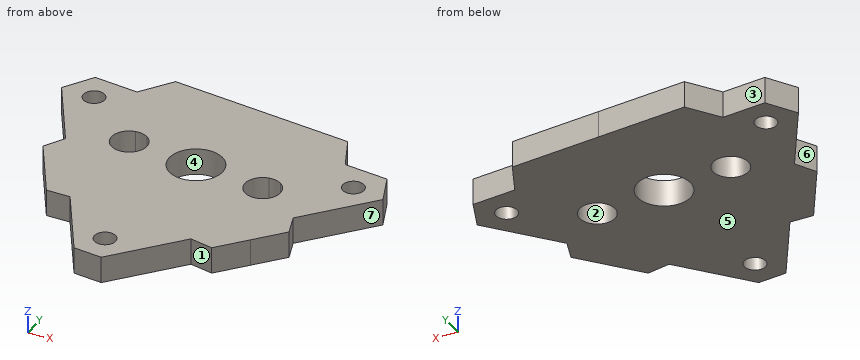
Autodesk Inventor part; units mm, degrees
ref_plane "YZ Plane" through (0, 0, 0) normal (1, 0, 0) x (0, 1, 0)
ref_plane "XZ Plane" through (0, 0, 0) normal (0, 1, 0) x (-1, 0, 0)
ref_plane "XY Plane" through (0, 0, 0) normal (0, 0, 1) x (1, 0, 0)
sketch "Sketch1" plane through (0, 0, 0) normal (0, 0, 1) x (1, 0, 0)
  circle A0 centre (-29.1799, 3.0736) radius 3.175 construction
  circle A1 centre (1.7526, 0) radius 3.175 construction
  circle A2 centre (-15.8567, -20.0304) radius 3.175 construction
  circle A3 centre (-29.1799, 3.0736) radius 1.2
  circle A4 centre (1.7526, 0) radius 1.2
  circle A5 centre (-15.8567, -20.0304) radius 1.2
  line L0 (-29.1799, 3.0736) -> (1.7526, 0) construction
  line L1 (-13.7137, 1.5368) -> (-15.8567, -20.0304) construction
  line L2 (-30.7954, 6.4247) -> (3.9959, 2.9677)
  line L3 (3.9959, 2.9677) -> (5.4173, -0.6401)
  line L4 (5.4173, -0.6401) -> (-14.5484, -23.3511)
  line L5 (-14.5484, -23.3511) -> (-17.7927, -23.0287)
  line L6 (-17.7927, -23.0287) -> (-32.899, 3.1671)
  line L7 (-32.899, 3.1671) -> (-30.7954, 6.4247)
  point P0 (0, 0)
  point P1 (-16.1706, -23.1899)
  point P2 (-31.8472, 4.7959)
  dimension "d0" = 2.4
  dimension "d1" = 2.4
  dimension "d2" = 2.4
extrude "Plate1" add sketch "Sketch1" along normal blind 3
sketch "Sketch2" plane through (0, 0, 3) normal (0, 0, 1) x (1, 0, 0)
  line L0 (-17.7927, -23.0287) -> (-32.899, 3.1671) construction
  line L1 (-30.7954, 6.4247) -> (3.9959, 2.9677) construction
  line L2 (5.4173, -0.6401) -> (-14.5484, -23.3511) construction
  line L3 (-17.7927, -23.0287) -> (-32.899, 3.1671) construction
  line L4 (-25.3459, -9.9308) -> (-14.2154, -3.5122) construction
  line L5 (-14.2154, -3.5122) -> (-13.3997, 4.6962) construction
  line L6 (-14.2154, -3.5122) -> (-4.5656, -11.9956) construction
  line L7 (5.4173, -0.6401) -> (-14.5484, -23.3511) construction
  point P0 (0, 0)
sketch "Sketch3" plane through (0, 0, 3) normal (0, 0, 1) x (1, 0, 0)
  arc A0 (-5.0898, -2.6774) -> (-6.5829, -2.3304) centre (-6.2546, -4.3032) ccw
  arc A1 (-6.5829, -2.3304) -> (-5.0898, -2.6774) centre (-6.2546, -4.3032) ccw
  arc A2 (-21.0113, -1.0954) -> (-22.5045, -0.7484) centre (-22.1762, -2.7212) ccw
  arc A3 (-22.5045, -0.7484) -> (-21.0113, -1.0954) centre (-22.1762, -2.7212) ccw
  circle A4 centre (-14.2154, -3.5122) radius 3
extrude "Extrusion1" cut sketch "Sketch3" against normal through all
sketch "Sketch4" plane through (0, 0, 0) normal (0, 0, -1) x (-1, 0, 0)
  line L0 (30.7954, 6.4247) -> (-3.9959, 2.9677)
  line L1 (0.9857, 3.4627) -> (2.77, 7.4096)
  line L2 (2.77, 7.4096) -> (13.0288, 8.429)
  line L3 (13.0288, 8.429) -> (13.3997, 4.6962) construction
  arc A0 (9.3955, 4.3921) -> (1.4831, 3.2621) centre (5.4635, 3.6576) ccw construction
  line L4 (25.8137, 5.9297) -> (23.2877, 9.4483)
  line L5 (23.2877, 9.4483) -> (13.0288, 8.429)
  line L6 (-5.4173, -0.6401) -> (14.5484, -23.3511)
  line L7 (0.9442, -7.8763) -> (0.0881, -10.4082)
  line L8 (0.0881, -10.4082) -> (2.8272, -13.5239)
  line L9 (2.8272, -13.5239) -> (4.5656, -11.9956) construction
  line L10 (-5.4173, -0.6401) -> (14.5484, -23.3511)
  arc A1 (3.0652, -12.6595) -> (11.0452, -12.2104) centre (7.0456, -12.264) ccw construction
  line L11 (8.1869, -16.1149) -> (5.5662, -16.6395)
  line L12 (5.5662, -16.6395) -> (2.8272, -13.5239)
  line L13 (17.7927, -23.0287) -> (32.899, 3.1671)
  line L14 (28.0858, -5.1794) -> (29.4234, -7.4934)
  line L15 (29.4234, -7.4934) -> (27.351, -11.0871)
  line L16 (25.2786, -14.6808) -> (27.351, -11.0871)
  line L17 (22.6059, -14.6822) -> (25.2786, -14.6808)
  point P0 (0, 0)
  dimension "d6" = 120
  dimension "d7" = 120
extrude "Extrusion2" add sketch "Sketch4" against normal up to surface (3 mm away)
equation "\"d3\" = Thickness"
equation "\"BendRadius\" = Thickness"
equation "\"BendReliefWidth\" = Thickness"
equation "\"BendReliefDepth\" = 0.5 * Thickness"
equation "\"CornerReliefSize\" = 4 * Thickness"
equation "\"MinimumRemnant\" = 2 * Thickness"
equation "\"TransitionRadius\" = BendRadius"
equation "\"JacobiRadiusSize\" = BendRadius"
equation "\"GapSize\" = Thickness"
properties part number "TongueMount"
Here's how the part is built. I have some questions about the finished solid (model axes, mm). Face numbers are marked on the shaded views. A direction names the side the tool comes from. Give positions to 0.01 mm unless a question says otherwise; leave off trailing zeros. Loops run counter-clockwise (first coordinate to the right, second up) from the corner with the lowest first, then second, coordinate; pieces in that order, holes last. Notation, with made-up numbers: (18, 65) -> (69, 65) arc R13 ccw to (69, 85) -> close; hole circle Ø10 at (27, 77). An arc over 180 degrees is marked (long way). Use one line per item in the form item = value. Start each with the question number.
1) Imagine slicing it at C-C (x = 1). Please give me the cut outline in (y, z), then the cut area to 3 significant figures.
2) Thinking about a two-plate mould opening in X: for the marked faces 4, 5, 6 and 7, which applies, +X half, -X half, draft (parallel to the pull), parting line (faces both ways), or undercut?
3) Imagine slicing it at A-A (y = 0). Please give me the cut outline in (x, z).
4) Which directions (+Z, -Z, +X, -X, +Y, -Y) give clear straight access to the entire face, cutting with the end or side of a thin tool? Please do the marked faces 1, 2 and 3.
5) Imagine slicing it at B-B (z = 0.9). Please give me the cut outline in (x, y).
6) Please list where these lines run through material, in increasing order: line 1 along Y through (x, z) = (-15.5, 2); line 2 along X through (y, z) = (-2.5, 0.2); line 3 along X through (y, z) = (-4.5, 1.15).
7) For P1, Ø1, axis at x = -18.5, z = 2.5, coming from the -Y side; P2, Ø5, axis at x = -22.18, y = -2.72, coming from the +Z side; P3, Ø1.9, axis at x = 1.75, y = 0, coming from the +Z side, each with a flat end and sliding along its axis, tell me the tip position at first contact or that it passes through.
8) Imagine slicing it at D-D (y = 7). Please give me the cut outline in (x, z), then the cut area to 3 significant figures.
Check values:
q1.outline = (-5.66, 0) -> (-0.93, 0) -> (-0.93, 3) -> (-5.66, 3) -> close; (0.93, 0) -> (3.27, 0) -> (3.27, 3) -> (0.93, 3) -> close
q1.area = 21.2 mm^2
q2.face_4 = undercut
q2.face_5 = draft
q2.face_6 = -X half
q2.face_7 = +X half
q3.outline = (-31.07, 0) -> (0.55, 0) -> (0.55, 3) -> (-31.07, 3) -> close; (2.95, 0) -> (5.17, 0) -> (5.17, 3) -> (2.95, 3) -> close
q4.face_1 = +Z, -Z, -Y
q4.face_2 = +Z, -Z
q4.face_3 = +Z, -Z, +Y
q5.outline = (-32.9, 3.17) -> (-28.09, -5.18) -> (-29.42, -7.49) -> (-25.28, -14.68) -> (-22.61, -14.68) -> (-17.79, -23.03) -> (-14.55, -23.35) -> (-8.19, -16.11) -> (-5.57, -16.64) -> (-2.83, -13.52) -> (-0.09, -10.41) -> (-0.94, -7.88) -> (5.42, -0.64) -> (4, 2.97) -> (-0.99, 3.46) -> (-2.77, 7.41) -> (-13.03, 8.43) -> (-23.29, 9.45) -> (-25.81, 5.93) -> (-30.8, 6.42) -> close; hole circle Ø2.4 at (-29.18, 3.07); hole (-22.5, -0.75) arc R2 ccw (long way) to (-21.01, -1.1) arc R2 ccw to start; hole circle Ø6 at (-14.22, -3.51); hole circle Ø2.4 at (-15.86, -20.03); hole (-6.58, -2.33) arc R2 ccw (long way) to (-5.09, -2.68) arc R2 ccw to start; hole circle Ø2.4 at (1.75, 0)
q6.line_1 = -23.26 to -21.18, -18.88 to -6.22, -0.8 to 8.67
q6.line_2 = -29.63 to -24.16, -20.19 to -17.04, -11.39 to -7.12, -5.39 to 3.78
q6.line_3 = -28.48 to -23.09, -21.26 to -17.05, -11.38 to -8.24, -4.26 to 2.02
q7.P1 = -22.67
q7.P2 = 3
q7.P3 = through
q8.outline = (-25.05, 0) -> (-2.58, 0) -> (-2.58, 3) -> (-25.05, 3) -> close
q8.area = 67.4 mm^2
